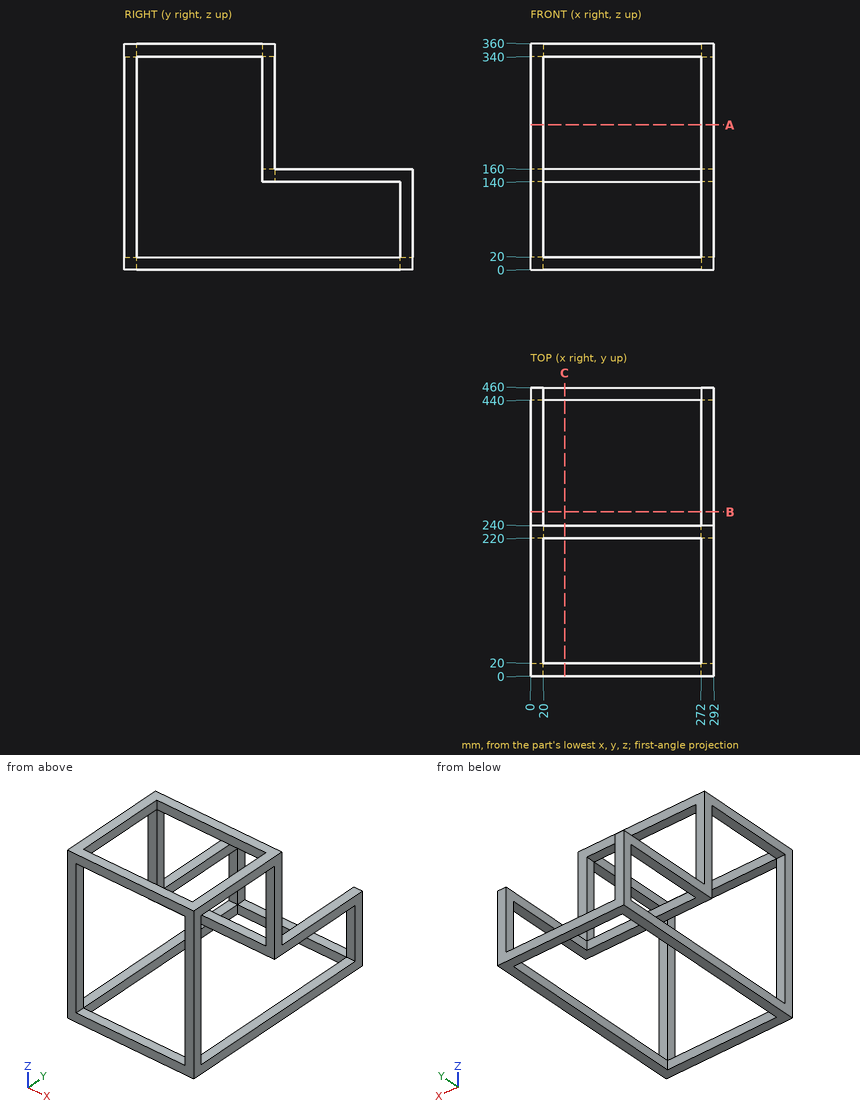
Geometry check sheet. Reference: drawing and pictorial views, mm from the part's lowest x, y, z. Round coordinates to 2 decimals unless told otherwise and drop trailing zeros. Order: outer loops, then holes, each group sorted by start corner. A loop starts at its lowest first (then second) coordinate and runs counter-clockwise, first axis right, second up. Notation, with made-up numbers: (54.25, 13.25) -> (69.25, 13.25) arc R13 ccw to (69.25, 30.25) -> close; hole circle Ø11 at (64, 28). An arc over 180 degrees is marked (long way). One line per item, written item: value. Start each with the question number.
Q1. Thickness scan on line 1 (X direction, y = 424, z = 142); line 2 (Y direction, x = 14, z = 113); line 3 (Y direction, x = 16.5, z = 342.5). Record the ranges inside material, lowest first.
Q2. Cross-section at C-C (x = 54). Record the boundary of the cut face in (y, z).
Q3. Gauge pin test, flat ends, axial feed: pin 1 Ø6 at (y, z) = (14, 110.5) entering from -X; pin 2 Ø4 at (x, z) = (105, 156.5) entering from -Y; pin 3 Ø16 at (x, y) = (174, 445.5) entering from +Z. Record the tip position at first contact, or that the pin passes through.
Q4. Cross-section at B-B (y = 262). Record the boundary of the cut face in (x, z).
Q5. Cross-section at A-A (z = 231). Record the boundary of the cut face in (x, y), and give its area (3 significant figures).
Completed:
1. line 1: x = 0 to 20, 272 to 292
1. line 2: y = 0 to 20, 440 to 460
1. line 3: y = 0 to 240
2. outline: (0, 0) -> (20, 0) -> (20, 20) -> (0, 20) -> close; (0, 340) -> (20, 340) -> (20, 360) -> (0, 360) -> close; (220, 140) -> (240, 140) -> (240, 160) -> (220, 160) -> close; (220, 340) -> (240, 340) -> (240, 360) -> (220, 360) -> close; (440, 0) -> (460, 0) -> (460, 20) -> (440, 20) -> close
3. pin 1: stops at x = 0
3. pin 2: stops at y = 220
3. pin 3: stops at z = 20
4. outline: (0, 0) -> (20, 0) -> (20, 20) -> (0, 20) -> close; (0, 140) -> (20, 140) -> (20, 160) -> (0, 160) -> close; (272, 0) -> (292, 0) -> (292, 20) -> (272, 20) -> close; (272, 140) -> (292, 140) -> (292, 160) -> (272, 160) -> close
5. outline: (0, 0) -> (20, 0) -> (20, 20) -> (0, 20) -> close; (0, 220) -> (20, 220) -> (20, 240) -> (0, 240) -> close; (272, 0) -> (292, 0) -> (292, 20) -> (272, 20) -> close; (272, 220) -> (292, 220) -> (292, 240) -> (272, 240) -> close
5. area: 1,600 mm²
